Can you work these out from the model? Positions are in its coordinate system, mm. Face numbers are marked on the shaded views. A direction names the side the tool comes from. Round coordinates to 2 decimals unless told otherwise and drop trailing zeros. Write each loop counter-clockwise with the first axis right and the second up, starting at its lowest first coordinate (ties: lowest second). Pieces come first, ordered by that corner, then holes. Notation, with made-up numbers: (15.5, 8) -> (42.5, 8) arc R34 cw to (42.5, 40) -> close; hole circle Ø2 at (13.25, 8.5). An arc over 180 degrees is marked (long way). Use CSV: the item, a comma, the result in double quotes.
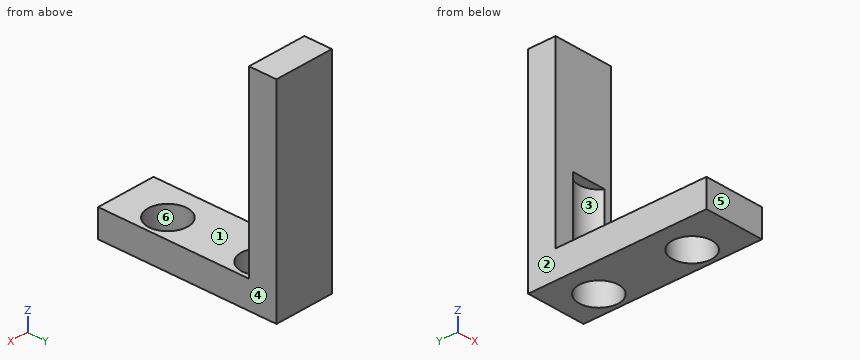
```python
from build123d import *

# Parameters (mm, degrees)
SKETCH1_W           = 6.5
SKETCH1_H           = 19.5
BOSS_EXTRUDE1_DEPTH = 3
SKETCH6_W           = 6.5
SKETCH6_H           = 19.754729726
BOSS_EXTRUDE2_DEPTH = 3
SKETCH7_R           = 2.15
CUT_EXTRUDE1_DEPTH  = 11


with BuildPart() as part:
    # Sketch1 → Boss-Extrude1 (new body)
    with BuildSketch(Plane.XY):
        with Locations((-30.832629628, -16.171363726)):
            Rectangle(SKETCH1_W, SKETCH1_H)
    extrude(amount=BOSS_EXTRUDE1_DEPTH)

    # Sketch6 → Boss-Extrude2 (add)
    with BuildSketch(Plane(origin=(0, -6.421363726, 0), x_dir=(1, 0, 0), z_dir=(0, 1, 0))):
        with Locations((-30.832629628, -12.877364863)):
            Rectangle(SKETCH6_W, SKETCH6_H)
    extrude(amount=-BOSS_EXTRUDE2_DEPTH)

    # Sketch7 → Cut-Extrude1 (cut)
    with BuildSketch(Plane(origin=(0, 0, 0), x_dir=(-1, 0, 0), z_dir=(0, 0, -1))):
        with Locations((30.182629628, -10.521084151)):
            Circle(SKETCH7_R)
        with Locations((30.182629628, -20.721084151)):
            Circle(SKETCH7_R)
    extrude(amount=-CUT_EXTRUDE1_DEPTH, mode=Mode.SUBTRACT)


solid = part.part
```
Q1. On a 3-axis mill with a long thin cutter (end or side, diameter ignored), from which of +Z, -Z, +X, -X, +Y, -Y can I reach the whole of each face in a straight line? I mean the marked faces 1, 2 and 3. Say none if no direction works.
Resolved:
face 1,"+Z, +X, -X, -Y"
face 2,"+Z, -Z, -X, +Y, -Y"
face 3,"-Z"
Q2. Suppose I cut it at C-C (z = 3.5). Write out the boundary of the cut face in (x, y), and give its area (3 significant figures).
Resolved:
outline,"(-34.08, -9.42) -> (-32.03, -9.42) arc R2.15 cw to (-28.34, -9.42) -> (-27.58, -9.42) -> (-27.58, -6.42) -> (-34.08, -6.42) -> close"
area,"16.8 mm^2"
Q3. Suppose I cut it at D-D (x = -33.25). Write out the boundary of the cut face in (y, z).
Resolved:
outline,"(-25.92, 0) -> (-6.42, 0) -> (-6.42, 22.75) -> (-9.42, 22.75) -> (-9.42, 3) -> (-25.92, 3) -> close"
Q4. Suppose I cut it at A-A (y = -11). Write out the boundary of the cut face in (x, z).
Resolved:
outline,"(-34.08, 0) -> (-32.28, 0) -> (-32.28, 3) -> (-34.08, 3) -> close; (-28.09, 0) -> (-27.58, 0) -> (-27.58, 3) -> (-28.09, 3) -> close"
Q5. Suppose I cut it at B-B (x = -29.75). Write out the boundary of the cut face in (y, z), and give its area (3 significant figures).
Resolved:
outline,"(-25.92, 0) -> (-22.83, 0) -> (-22.83, 3) -> (-25.92, 3) -> close; (-18.62, 0) -> (-12.63, 0) -> (-12.63, 3) -> (-18.62, 3) -> close; (-9.42, 11) -> (-8.42, 11) -> (-8.42, 0) -> (-6.42, 0) -> (-6.42, 22.75) -> (-9.42, 22.75) -> close"
area,"84.4 mm^2"
Q6. Please list where these lines run through material, in increasing order: probe 1 along Y at (x, z) = (-28.5, 18); probe 2 along Z at (x, y) = (-32.75, -19.5); probe 3 along X at (y, z) = (-9.25, 1.5).
Resolved:
probe 1,"y = -9.42 to -6.42"
probe 2,"z = 0 to 3"
probe 3,"x = -34.08 to -31.92, -28.45 to -27.58"
Q7. If we mould it in two halves opening along X, with no side actions, what happens to the marked faces 4, 5 and 6? For each: released by +X, released by -X, zero draft, split by the parting line, or undercut.
Resolved:
face 4,"released by +X"
face 5,"zero draft"
face 6,"undercut"
Q8. Will this pin go through, and if not, where does the flat tip stop? P1, Ø2, axis at x = -32, y = -18, coming from the +Z side.
Resolved:
P1,"stops at z = 3"
